Source: CAD feature listing. Evaluate the final solid. Frame: model axes, mm. A direction names the side the tool comes from. Give positions to 0.01 mm unless a question says otherwise; leave off trailing zeros. Write each loop counter-clockwise with the first axis right and the second up, starting at its lowest first coordinate (ties: lowest second). Pieces come first, ordered by that corner, then holes. Notation, with made-up numbers: M -14,-19.5 L 21,-19.5 A35 cw 21,19.5 Z; hole C 25,-9 d10. An arc over 180 degrees is marked long. Use CSV: the item, a comma, the result in double quotes. Start each with the question number.
from build123d import *

# Parameters (mm, degrees)
SKETCH1_R           = 4.7625
BOSS_EXTRUDE1_DEPTH = 3.175
SKETCH2_R           = 2.54
BOSS_EXTRUDE2_DEPTH = 3.81
SKETCH3_R           = 2.413
BOSS_EXTRUDE3_DEPTH = 6.35
CHAMFER1_SIZE       = 0.508
SKETCH8_W           = 0.635
SKETCH8_H           = 1.27
CHAMFER2_SIZE       = 0.762


with BuildPart() as part:
    # Sketch1 → Boss-Extrude1 (new body)
    with BuildSketch(Plane.XY):
        Circle(SKETCH1_R)
    extrude(amount=BOSS_EXTRUDE1_DEPTH)

    # Sketch2 → Boss-Extrude2 (add)
    with BuildSketch(Plane.XY.offset(3.175)):
        Circle(SKETCH2_R)
    extrude(amount=BOSS_EXTRUDE2_DEPTH)

    # Sketch3 → Boss-Extrude3 (add)
    with BuildSketch(Plane.XY.offset(6.985)):
        Circle(SKETCH3_R)
    extrude(amount=BOSS_EXTRUDE3_DEPTH)

    # Chamfer1
    chamfer1_edges = [part.edges().sort_by_distance(p)[0] for p in [
        (-2.413, 0, 13.335),
    ]]
    chamfer(chamfer1_edges, length=CHAMFER1_SIZE)

    # Sketch8 → Cut-Revolve1 (revolve, cut)
    with BuildSketch(Plane(origin=(0, 0, 0), x_dir=(1, 0, 0), z_dir=(0, 1, 0))):
        with Locations((-2.2225, -7.62)):
            Rectangle(SKETCH8_W, SKETCH8_H)
    revolve(axis=Axis((0, 0, 23.053781971), (0, 0, -1)), mode=Mode.SUBTRACT)

    # Chamfer2
    chamfer2_edges = [part.edges().sort_by_distance(p)[0] for p in [
        (-4.7625, 0, 0),
        (-4.7625, 0, 3.175),
    ]]
    chamfer(chamfer2_edges, length=CHAMFER2_SIZE)


solid = part.part
Item 1: Section A-A (x = 0). Return the cut outline in (y, z) (1 decimal), plus the area to 3 significant figures.
Item 2: Section C-C (z = 3.75). Return the cut outline in (x, y), plus the area to 3 significant figures.
Item 3: Section D-D (z = 11). Return the cut outline in (x, y), plus the area to 3 significant figures.
Item 4: Pull-direction query (Z, two-part tool) for faces 4 (the flat face through (-2, 1, 8.255)), 5 (the flat face through (1, 2, 6.985)), 6 (the flat face through (0, 0, 13.335)), 7 (the cylindrical face through (-0.33, 2.52, 5.05)); classes: released by +Z, released by -Z, zero draft, split by the parting line, or undercut.
Item 5: Material intervals for probe 1 along Z at (x, y) = (0, -2.5) (3 decimals); probe 2 along Z at (x, y) = (-1, 2.5) (3 decimals); probe 3 along Y at (x, z) = (1, 3.25), sorted ascending.
Item 6: Set-up query: faces 1 (the flat face through (0, 0, 0)), 2 (the cylindrical face through (0.41, -1.86, 7.61)), 3 (the cylindrical face through (-1.915, -1.468, 10.509)). Return all of +Z, -Z, +X, -X, +Y, -Y with unobstructed straight access to the full face (end or side cutting, diameter ignored); none if empty.
Output values:
1,outline,"M -4.8,0.8 L -4,0 L 4,0 L 4.8,0.8 L 4.8,2.4 L 4,3.2 L 2.5,3.2 L 2.5,7 L 1.9,7 L 1.9,8.3 L 2.4,8.3 L 2.4,12.8 L 1.9,13.3 L -1.9,13.3 L -2.4,12.8 L -2.4,8.3 L -1.9,8.3 L -1.9,7 L -2.5,7 L -2.5,3.2 L -4,3.2 L -4.8,2.4 Z"
1,area,"77.5 mm2"
2,outline,"C 0,0 d5.08"
2,area,"20.3 mm2"
3,outline,"C 0,0 d4.83"
3,area,"18.3 mm2"
4,face 4,"undercut"
4,face 5,"undercut"
4,face 6,"released by +Z"
4,face 7,"zero draft"
5,probe 1,"z = 0 to 6.985"
5,probe 2,"z = 0 to 3.175"
5,probe 3,"y = -2.33 to 2.33"
6,face 1,"-Z, +X, -X, +Y, -Y"
6,face 2,"none"
6,face 3,"+Z"
